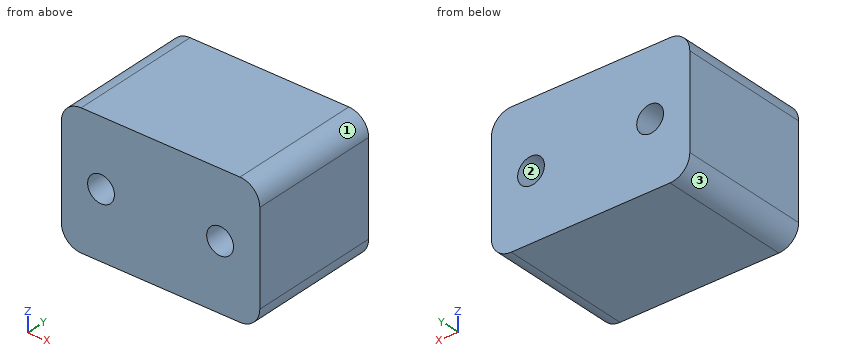
from build123d import *

# Parameters (mm, degrees)
SKETCH_1_W          = 30
SKETCH_1_H          = 20
EXTRUDE_1_DEPTH     = 20
SKETCH_2_R          = 2.025
CUT_EXTRUDE_1_DEPTH = 20
FILLET_1_R          = 3


with BuildPart() as part:
    # 草图1 → 凸台-拉伸1 (new body)
    with BuildSketch(Plane(origin=(0, 0, 0), x_dir=(1, 0, 0), z_dir=(0, 1, 0))):
        Rectangle(SKETCH_1_W, SKETCH_1_H)
    extrude(amount=EXTRUDE_1_DEPTH)

    # 草图2 → 切除-拉伸1 (cut)
    with BuildSketch(Plane(origin=(0, 20, 0), x_dir=(1, 0, 0), z_dir=(0, 1, 0))):
        with Locations((-9, 0)):
            Circle(SKETCH_2_R)
        with Locations((9, 0)):
            Circle(SKETCH_2_R)
    extrude(amount=-CUT_EXTRUDE_1_DEPTH, mode=Mode.SUBTRACT)

    # 圆角1
    fillet_1_edges = [part.edges().sort_by_distance(p)[0] for p in [
        (15, 10, 10),
        (-15, 10, 10),
        (-15, 10, -10),
        (15, 10, -10),
    ]]
    fillet(fillet_1_edges, radius=FILLET_1_R)


solid = part.part
The listing builds one solid part. Answer for the finished solid, in the listing's coordinates (mm). Face numbers are marked on the shaded views. Coordinates: 2 decimals unless noted, no trailing zeros. Loops run counter-clockwise (first coordinate to the right, second up) from the corner with the lowest first, then second, coordinate; pieces in that order, holes last.
1) Find section B-B on x = 9. Write down the section's boundary in (y, z) (3 decimals).
2) Find section A-A on z = 0. Write down the section's boundary in (x, y) (3 decimals), then the cut area to 3 significant figures.
3) Find the intervals of material crossed by L1, parallel to X at y = 11.5, z = 0 (3 decimals); L2, parallel to Z at x = -9, y = 14.25 (3 decimals); L3, parallel to X at y = 3.75, z = 8.5, in increasing order.
4) Find section C-C on y = 9.75. Write down the section's boundary in (x, z) (3 decimals), then the cut area to 3 significant figures.
5) Determine the mould class of the marked faces 1, 2 and 3 for opening direction X: pulls with the +X half, pulls with the -X half, needs draft (parallel to the pull), parting line crosses it, or undercut.
6) A flat-ended cylindrical pin translates along its axis: pin 1 Ø2.5 at (x, z) = (9, 0) entering from -Y. Find the tip coordinate at first contact, or state that the pin passes through.
Values:
1. outline: (0, -10) - (20, -10) - (20, -2.025) - (0, -2.025) - close; (0, 2.025) - (20, 2.025) - (20, 10) - (0, 10) - close
2. outline: (-15, 0) - (-11.025, 0) - (-11.025, 20) - (-15, 20) - close; (-6.975, 0) - (6.975, 0) - (6.975, 20) - (-6.975, 20) - close; (11.025, 0) - (15, 0) - (15, 20) - (11.025, 20) - close
2. area: 438 mm2
3. L1: x = -15 to -11.025, -6.975 to 6.975, 11.025 to 15
3. L2: z = -10 to -2.025, 2.025 to 10
3. L3: x = -14.6 to 14.6
4. outline: (-15, -7) arc R3 ccw to (-12, -10) - (12, -10) arc R3 ccw to (15, -7) - (15, 7) arc R3 ccw to (12, 10) - (-12, 10) arc R3 ccw to (-15, 7) - close; hole circle Ø4.05 at (-9, 0); hole circle Ø4.05 at (9, 0)
4. area: 567 mm2
5. face 1: pulls with the +X half
5. face 2: undercut
5. face 3: pulls with the -X half
6. pin 1: passes through
